Here's the drawing with two shaded views (mm, measured from the low corner). I have some questions. A direction names the side the tool comes from. Round coordinates to 2 decimals unless told otherwise and drop trailing zeros. Loops run counter-clockwise (first coordinate to the right, second up) from the corner with the lowest first, then second, coordinate; pieces in that order, holes last.
(1) I want a section at D-D on x = 25. Write out the boundary of the cut face in (y, z), plus the area to 3 significant figures.
(2) Will these pins go through, and if not, where does the flat tip stop? pin 1 Ø5 at (x, y) = (24, 7.5) entering from +Z; pin 2 Ø4 at (x, z) = (45.5, 28) entering from -Y; pin 3 Ø5 at (x, y) = (80.5, 9) entering from +Z; pin 4 Ø12 at (x, z) = (84, 25) entering from -Y.
(3) Thinking about a two-plate mould opening in Z: for the marked faces 1, 2, 3 and 4, which applies, released by +Z, released by -Z, zero draft, split by the parting line, or undercut?
(4) Which directions (+Z, -Z, +X, -X, +Y, -Y) give clear straight access to the entire face, cutting with the end or side of a thin tool? Please do the marked faces 5, 6, 7 and 8.
(5) I want a section at C-C on x = 84. Write out the boundary of the cut face in (y, z), plus the area to 3 significant figures.
(6) I want a section at A-A on y = 7. Write out the boundary of the cut face in (x, z), plus the area to 3 significant figures.
(7) If I drill on line 1 along Z through (x, y) = (84, 16.3); line 2 along Z through (x, y) = (25, 16.3); line 3 along Z through (x, y) = (84, 10), over which ranges is the centre line in solid material (lowest first)?
(8) I want a section at B-B on z = 25. Write out the boundary of the cut face in (x, y).
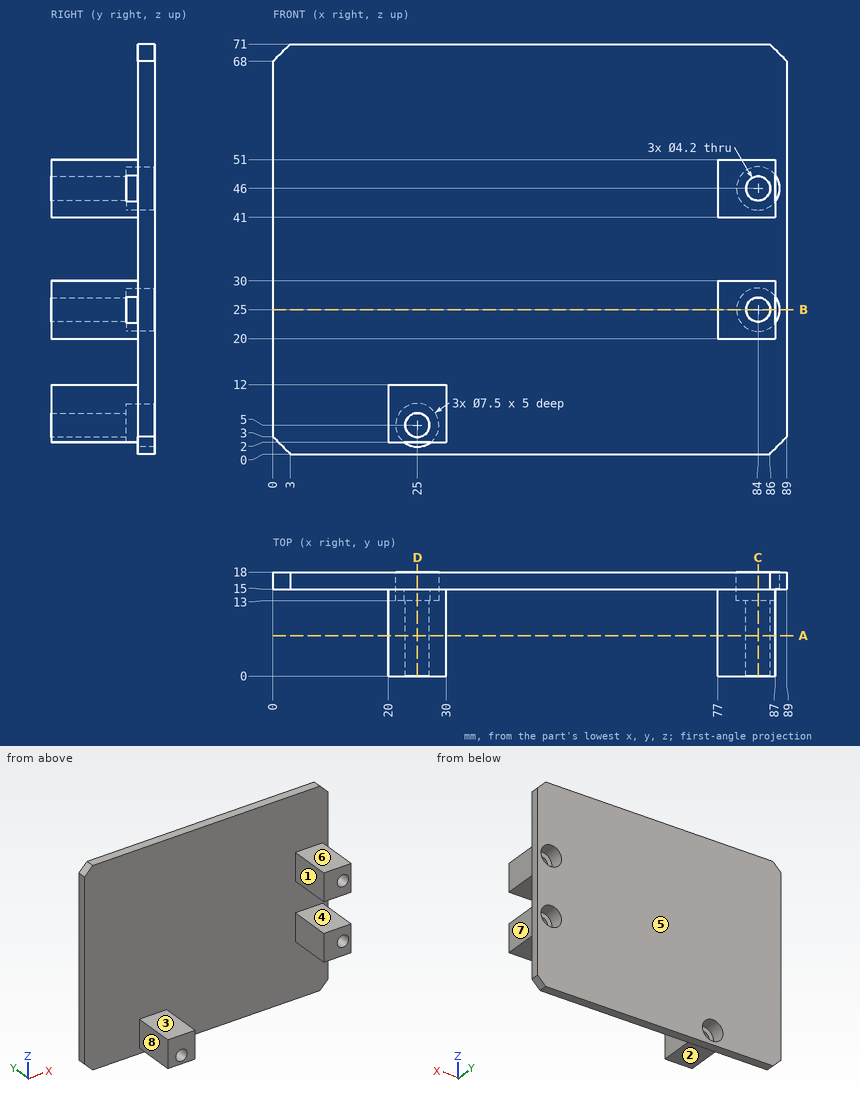
Filled sheet:
1. outline: (0, 2) - (13, 2) - (13, 2.9) - (0, 2.9) - close; (0, 7.1) - (13, 7.1) - (13, 8.75) - (18, 8.75) - (18, 71) - (15, 71) - (15, 12) - (0, 12) - close; (15, 0) - (18, 0) - (18, 1.25) - (15, 1.25) - close
1. area: 272 mm2
2. pin 1: stops at z = 12
2. pin 2: stops at y = 15
2. pin 3: stops at z = 51
2. pin 4: stops at y = 0
3. face 1: zero draft
3. face 2: released by -Z
3. face 3: released by +Z
3. face 4: undercut
4. face 5: +Z, -Z, +X, -X, +Y
4. face 6: +Z, +X, -X, -Y
4. face 7: +Z, -Z, +X, -Y
4. face 8: +Z, -Z, -X, -Y
5. outline: (0, 20) - (15, 20) - (15, 0) - (18, 0) - (18, 21.25) - (13, 21.25) - (13, 22.9) - (0, 22.9) - close; (0, 27.1) - (13, 27.1) - (13, 28.75) - (18, 28.75) - (18, 42.25) - (13, 42.25) - (13, 43.9) - (0, 43.9) - (0, 41) - (15, 41) - (15, 30) - (0, 30) - close; (0, 48.1) - (13, 48.1) - (13, 49.75) - (18, 49.75) - (18, 71) - (15, 71) - (15, 51) - (0, 51) - close
5. area: 329 mm2
6. outline: (20, 2) - (30, 2) - (30, 12) - (20, 12) - close; (77, 20) - (87, 20) - (87, 30) - (77, 30) - close; (77, 41) - (87, 41) - (87, 51) - (77, 51) - close; hole circle Ø4.2 at (25, 5); hole circle Ø4.2 at (84, 25); hole circle Ø4.2 at (84, 46)
6. area: 258 mm2
7. line 1: z = 0 to 21.25, 28.75 to 42.25, 49.75 to 71
7. line 2: z = 0 to 1.25, 8.75 to 71
7. line 3: z = 20 to 22.9, 27.1 to 30, 41 to 43.9, 48.1 to 51
8. outline: (0, 15) - (77, 15) - (77, 0) - (81.9, 0) - (81.9, 13) - (80.25, 13) - (80.25, 18) - (0, 18) - close; (86.1, 0) - (87, 0) - (87, 13) - (86.1, 13) - close; (87.75, 15) - (89, 15) - (89, 18) - (87.75, 18) - close
